```python
from build123d import *

# Parameters (mm, degrees)
BOSS_EXTRUDE1_DEPTH                                  = 20
CBORE_FOR_M3_HEXAGON_SOCKET_HEAD_CAP_SCR_D           = 3.2
CBORE_FOR_M3_HEXAGON_SOCKET_HEAD_CAP_SCR_CBORE_D     = 6
CBORE_FOR_M3_HEXAGON_SOCKET_HEAD_CAP_SCR_CBORE_DEPTH = 3.4
FILLET1_R                                            = 8
CHAMFER1_SIZE                                        = 20
M6_TAPPED_HOLE1_D                                    = 5
M6_TAPPED_HOLE1_CSINK_D                              = 6.05
M6_TAPPED_HOLE1_CSINK_ANGLE                          = 90
CHAMFER2_SIZE                                        = 5


with BuildPart() as part:
    # Sketch1 → Boss-Extrude1 (new body)
    with BuildSketch(Plane.XY):
        Polygon((0, 0), (-45, 0), (-45, -20), (20, -20), (20, 35), (0, 35), align=None)
    extrude(amount=BOSS_EXTRUDE1_DEPTH)

    # CBORE for M3 Hexagon socket head cap screws1 (through all)
    with Locations(Plane.XY.offset(20)):
        with Locations((-35, -10), (-20, -10), (10, 25), (10, 10)):
            CounterBoreHole(CBORE_FOR_M3_HEXAGON_SOCKET_HEAD_CAP_SCR_D / 2, CBORE_FOR_M3_HEXAGON_SOCKET_HEAD_CAP_SCR_CBORE_D / 2, CBORE_FOR_M3_HEXAGON_SOCKET_HEAD_CAP_SCR_CBORE_DEPTH)

    # Fillet1
    fillet1_edges = [part.edges().sort_by_distance(p)[0] for p in [
        (0, 0, 10),
    ]]
    fillet(fillet1_edges, radius=FILLET1_R)

    # Chamfer1
    chamfer1_edges = [part.edges().sort_by_distance(p)[0] for p in [
        (20, -20, 10),
    ]]
    chamfer(chamfer1_edges, length=CHAMFER1_SIZE)

    # M6 Tapped Hole1 (through all)
    with Locations(Plane(origin=(10, -10, 0), x_dir=(-0.7071067811865495, -0.7071067811865457, 0), z_dir=(0.7071067811865457, -0.7071067811865495, 0))):
        with Locations((0, -10)):
            CounterSinkHole(M6_TAPPED_HOLE1_D / 2, M6_TAPPED_HOLE1_CSINK_D / 2, counter_sink_angle=M6_TAPPED_HOLE1_CSINK_ANGLE)

    # Chamfer2
    chamfer2_edges = [part.edges().sort_by_distance(p)[0] for p in [
        (0, 21.5, 20),
        (-26.5, 0, 20),
        (-2.343145751, 2.343145751, 20),
    ]]
    chamfer(chamfer2_edges, length=CHAMFER2_SIZE)


solid = part.part
```
Model file for the job. Use its own axes, mm. A direction names the side the tool comes from. Coordinates: 2 decimals unless noted, no trailing zeros. Order: outer loops, then holes, each group sorted by start corner. A loop starts at its lowest first (then second) coordinate and runs counter-clockwise, first axis right, second up. Notation, with made-up numbers: M 88,30 L 128,30 A25 cw 128,60 Z; hole C 18,-28.5 d11. An arc over 180 degrees is marked long. Answer as CSV lines item,"result".
(1) 3-axis set-ups, long thin cutter, end or side, ignore diameter. For faces 4 (the flat face through (-3, -5, 20)), 5 (the cylindrical face through (-23, -10, 18)), 6 (the flat face through (2, 22, 17)): which of +Z, -Z, +X, -X, +Y, -Y reach the whole face in a straight line?
Geometry says:
face 4,"+Z, +X, -X, +Y, -Y"
face 5,"+Z"
face 6,"+Z, -X, +Y"
(2) Wall check: line 1 along Y through (x, z) = (-20, 4.75); line 2 along X through (y, z) = (-8, 17); line 3 along Y through (x, z) = (-40, 2). Give the ranges that are in metal, low to high.
Geometry says:
line 1,"y = -20 to -11.6, -8.4 to 0"
line 2,"x = -45 to -37.24, -32.76 to -22.24, -17.76 to 12"
line 3,"y = -20 to 0"
(3) Flat gauge pins, fed straight in: pin 1 (1.8 mm diameter, centred on x = -21, y = -9.5, fed in from +Z); pin 2 (12 mm diameter, centred on x = -31.5, z = 10, fed in from +Y); pin 3 (4.5 mm diameter, centred on y = 20.5, z = 5.5, fed in from -X). Where does each tip first touch, or does it go through?
Geometry says:
pin 1,"stops at z = 16.6"
pin 2,"stops at y = 0"
pin 3,"stops at x = 0"
(4) Pull direction Y, two halves, no side cores. Call faces 1 (the cylindrical face through (-33.73, -10.97, 8.18)), 2 (the flat face through (0, 22, 7)), 3 (the flat face through (-23, -20, 10)): +Y half, -Y half, draft (parallel to the pull), parting line (faces both ways), or undercut.
Geometry says:
face 1,"undercut"
face 2,"draft"
face 3,"-Y half"
(5) Band-saw the part on C-C, the plane z = 3.25. List the corners of the cut face in (x, y).
Geometry says:
outline,"M -45,-20 L 0,-20 L 20,0 L 20,35 L 0,35 L 0,8 A8 cw -8,0 L -45,0 Z; hole C -35,-10 d3.2; hole C -20,-10 d3.2; hole C 10,10 d3.2; hole C 10,25 d3.2"
(6) Band-saw the part on B-B, the plane x = -35. List the corners of the cut face in (y, z).
Geometry says:
outline,"M -20,0 L -11.6,0 L -11.6,16.6 L -13,16.6 L -13,20 L -20,20 Z; M -8.4,0 L 0,0 L 0,15 L -5,20 L -7,20 L -7,16.6 L -8.4,16.6 Z"
(7) Band-saw the part on D-D, the plane y = 30.5. List the corners of the cut face in (x, z).
Geometry says:
outline,"M 0,0 L 20,0 L 20,20 L 5,20 L 0,15 Z"
(8) Band-saw the part on A-A, the plane y = 10. List the corners of the cut face in (x, z), then the cut area to 3 significant figures.
Geometry says:
outline,"M 0,0 L 8.4,0 L 8.4,16.6 L 7,16.6 L 7,20 L 5,20 L 0,15 Z; M 11.6,0 L 20,0 L 20,20 L 13,20 L 13,16.6 L 11.6,16.6 Z"
area,"314 mm2"
